from build123d import *

# Parameters (mm, degrees)
F0_R          = 37.5
F0_R_2        = 35
F1_DEPTH      = 2
F1_DEPTH_BACK = 2
F2_R          = 37.5
F2_R_2        = 31
F3_DEPTH      = 2
F4_R          = 37.5
F4_R_2        = 31
F5_DEPTH      = 2


# Not quite as in the source:
# - a feature names something its author has since deleted; it is built from what else it names


with BuildPart() as f1:
    # F0 (on Front) → F1 (new body, two sides)
    with BuildSketch(Plane.XZ) as f1_sk:
        Circle(F0_R)
        Circle(F0_R_2, mode=Mode.SUBTRACT)
    extrude(amount=-F1_DEPTH)
    extrude(f1_sk.sketch, amount=F1_DEPTH_BACK)

    # F2 (on face) → F3 (join)
    with BuildSketch(Plane.XZ.offset(2)):
        Circle(F2_R)
        Circle(F2_R_2, mode=Mode.SUBTRACT)
    extrude(amount=F3_DEPTH)

    # F4 (on face) → F5 (join)
    with BuildSketch(Plane(origin=(0, 2, 0), x_dir=(-1, 0, 0), z_dir=(0, 1, 0))):
        Circle(F4_R)
        Circle(F4_R_2, mode=Mode.SUBTRACT)
    extrude(amount=F5_DEPTH)


solid = f1.part
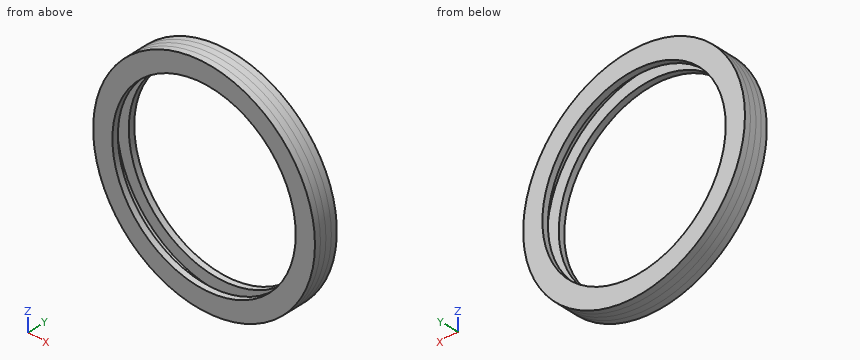
The listing builds one solid part. Answer for the finished solid, in the listing's coordinates (mm). Give positions to 0.01 mm unless a question says otherwise; leave off trailing zeros. Loops run counter-clockwise (first coordinate to the right, second up) from the corner with the lowest first, then second, coordinate; pieces in that order, holes last.
Item 1: A cutting plane is placed at B-B (z = 0). Give the vertices of the cut face in (x, y).
Derived:
outline: (-37.5, -4) - (-31, -4) - (-31, -2) - (-35, -2) - (-35, 2) - (-31, 2) - (-31, 4) - (-37.5, 4) - close; (31, -4) - (37.5, -4) - (37.5, 4) - (31, 4) - (31, 2) - (35, 2) - (35, -2) - (31, -2) - close
Item 2: A cutting plane is placed at A-A (x = 0). Give the vertices of the cut face in (y, z), then the cut area to 3 significant figures.
Derived:
outline: (-4, -37.5) - (4, -37.5) - (4, -31) - (2, -31) - (2, -35) - (-2, -35) - (-2, -31) - (-4, -31) - close; (-4, 31) - (-2, 31) - (-2, 35) - (2, 35) - (2, 31) - (4, 31) - (4, 37.5) - (-4, 37.5) - close
area: 72.0 mm2
Item 3: Find the intervals of material crossed by line 1 along Z through (x, y) = (0, -2.5); line 2 along Z through (x, y) = (0, 0.5); line 3 along Y through (x, z) = (1, 34.5), in increasing order.
Derived:
line 1: z = -37.5 to -31, 31 to 37.5
line 2: z = -37.5 to -35, 35 to 37.5
line 3: y = -4 to -2, 2 to 4
Item 4: A cutting plane is placed at C-C (z = -32.5). Give the vertices of the cut face in (x, y).
Derived:
outline: (-18.71, -4) - (18.71, -4) - (18.71, 4) - (-18.71, 4) - close; hole (-12.99, -2) - (12.99, -2) - (12.99, 2) - (-12.99, 2) - close
Item 5: Each of these flat-tipped pins is pushed along its axis until it touches: pin 1 Ø4 at (x, y) = (-18, 1.5) entering from +Z; pin 2 Ø4 at (y, z) = (-1.5, 17.5) entering from +X; pin 3 Ø2 at (y, z) = (2, -4.5) entering from +X. Where does it stop, or does it pass through?
Derived:
pin 1: stops at z = 33.92
pin 2: stops at x = 34.15
pin 3: stops at x = 37.34
Item 6: A cutting plane is placed at D-D (y = -1). Give the vertices of the cut face in (x, z), then the cut area to 3 significant figures.
Derived:
outline: circle Ø75 at (0, 0); hole circle Ø70 at (0, 0)
area: 569 mm2
